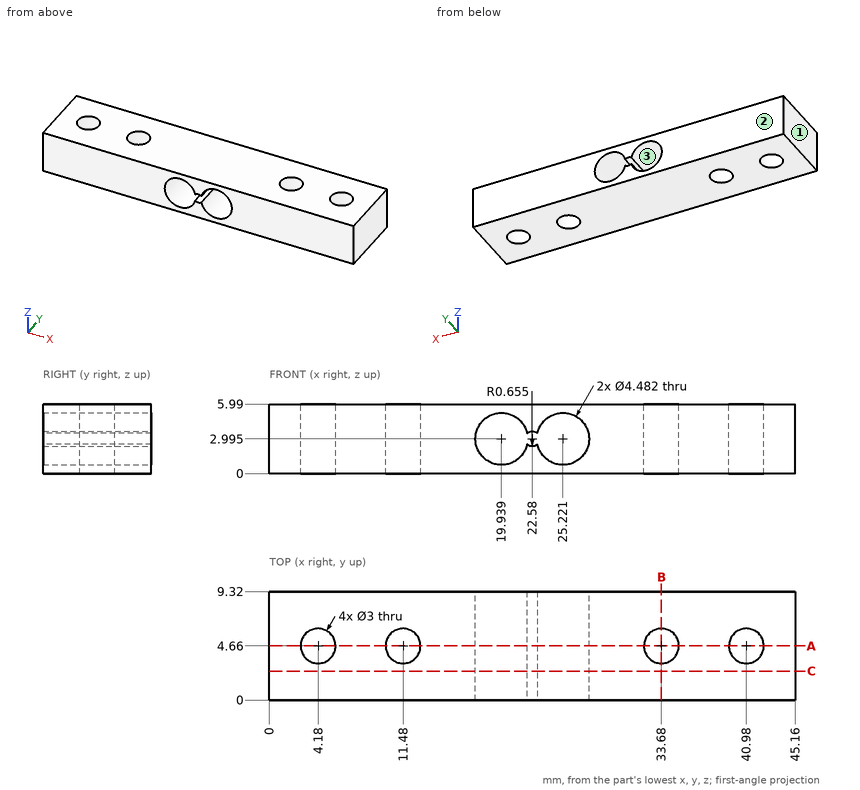
The drawing under review shows one solid part. Ordinate dimensions are in mm from its lowest x, y, z. Give positions to 0.01 mm unless a question says otherwise; leave off trailing zeros. Write each loop counter-clockwise with the first axis right and the second up, starting at its lowest first coordinate (ties: lowest second). Pieces come first, ordered by that corner, then holes. Notation, with made-up numbers: (65, 6.5) -> (86, 6.5) arc R32 cw to (86, 42.5) -> close; hole circle Ø11 at (0, 51.25). An arc over 180 degrees is marked (long way). Use CSV: the item, a comma, the result in double quotes.
Q1. For P1, Ø2.5, axis at x = 40.98, y = 4.66, coming from the +Z side; P2, Ø3.5, axis at x = 11.48, y = 4.66, coming from the -Z side, all flat-tipped, find the tip position at first contact; note any pin that passes through.
Conclusion:
P1,"through"
P2,"z = 0"
Q2. Take a section at B-B, the plane x = 33.68. Write out the cut boundary in (y, z).
Conclusion:
outline,"(0, 0) -> (3.16, 0) -> (3.16, 5.99) -> (0, 5.99) -> close; (6.16, 0) -> (9.32, 0) -> (9.32, 5.99) -> (6.16, 5.99) -> close"
Q3. Take a section at C-C, the plane y = 2.5. Write out the cut boundary in (x, z) (1 decimal).
Conclusion:
outline,"(0, 0) -> (45.2, 0) -> (45.2, 6) -> (0, 6) -> close; hole (22.1, 2.5) arc R0.7 ccw to (23, 2.5) arc R2.2 ccw (long way) to (23, 3.5) arc R0.7 ccw to (22.1, 3.5) arc R2.2 ccw (long way) to start"
Q4. To check wall thickness, follow probe 1 along X at (y, z) = (2, 3.1); probe 2 along Y at (x, z) = (4.18, 4.3); probe 3 along X at (y, z) = (7.25, 3.8). State the ranges of each line that lie inside material, in increasing order. Write a range as [from, to].
Conclusion:
probe 1,"[0, 17.7], [27.46, 45.16]"
probe 2,"[0, 3.16], [6.16, 9.32]"
probe 3,"[0, 17.85], [22.03, 23.13], [27.31, 45.16]"
Q5. Mouldability with a two-part tool opening along X and no side actions: class the marked faces 1, 2 and 3 as pulls with the +X half, pulls with the -X half, needs draft (parallel to the pull), parting line crosses it, or undercut.
Conclusion:
face 1,"pulls with the -X half"
face 2,"needs draft"
face 3,"undercut"
Q6. Take a section at A-A, the plane y = 4.66. Write out the cut boundary in (x, z) (1 decimal), then the cut area to 3 significant figures.
Conclusion:
outline,"(0, 0) -> (2.7, 0) -> (2.7, 6) -> (0, 6) -> close; (5.7, 0) -> (10, 0) -> (10, 6) -> (5.7, 6) -> close; (13, 0) -> (32.2, 0) -> (32.2, 6) -> (13, 6) -> close; (35.2, 0) -> (39.5, 0) -> (39.5, 6) -> (35.2, 6) -> close; (42.5, 0) -> (45.2, 0) -> (45.2, 6) -> (42.5, 6) -> close; hole (22.1, 2.5) arc R0.7 ccw to (23, 2.5) arc R2.2 ccw (long way) to (23, 3.5) arc R0.7 ccw to (22.1, 3.5) arc R2.2 ccw (long way) to start"
area,"166 mm2"
